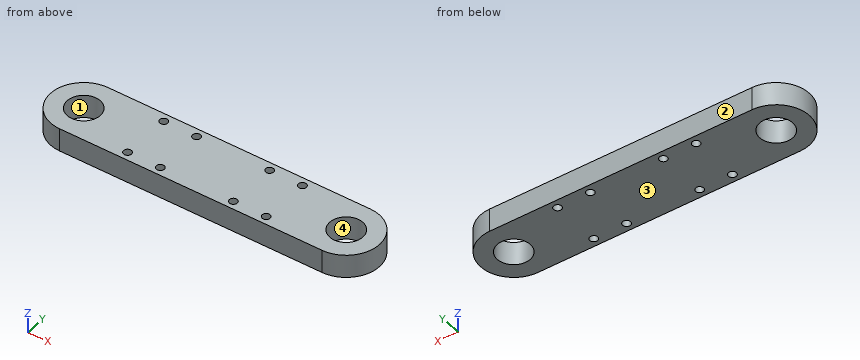
```python
from build123d import *

# Parameters (mm, degrees)
SKETCH_1_R          = 10
SKETCH_1_R_2        = 5
EXTRUDE_1_DEPTH     = 7
SKETCH_2_R          = 1.2
CUT_EXTRUDE_1_DEPTH = 10
CUT_EXTRUDE_START   = -10
SKETCH_3_R          = 5
CUT_EXTRUDE_2_DEPTH = 10
SKETCH_4_R          = 1.2
CUT_EXTRUDE_3_DEPTH = 10


with BuildPart() as part:
    # 草图1 → 凸台-拉伸1 (new body)
    # profile 1 of 2: a face of its own
    with BuildSketch(Plane.XY):
        Circle(SKETCH_1_R)
        Circle(SKETCH_1_R_2, mode=Mode.SUBTRACT)
    # profile 2 of 2: a face of its own
    with BuildSketch(Plane.XY):
        with BuildLine():
            Line((80, 10), (0, 10))
            ThreePointArc((0, 10), (7.071067812, 7.071067812), (10, 0))
            ThreePointArc((10, 0), (7.071067812, -7.071067812), (0, -10))
            Line((0, -10), (80, -10))
            ThreePointArc((80, -10), (90, 0), (80, 10))
        make_face()
    extrude(amount=EXTRUDE_1_DEPTH)

    # 草图2 → 切除-拉伸1 (cut)
    with BuildSketch(Plane(origin=(0, 0, 0), x_dir=(-1, 0, 0), z_dir=(0, 0, -1))):
        with Locations((-51.129038153, -7.5)):
            Circle(SKETCH_2_R)
        with Locations((-61.129038153, -7.5)):
            Circle(SKETCH_2_R)
        with Locations((-61.129038153, 7.5)):
            Circle(SKETCH_2_R)
        with Locations((-51.129038153, 7.5)):
            Circle(SKETCH_2_R)
    extrude(amount=-CUT_EXTRUDE_1_DEPTH, mode=Mode.SUBTRACT)

    # 草图3 → 切除-拉伸2 (cut)
    with BuildSketch(Plane.XY.offset(7).offset(CUT_EXTRUDE_START)):
        Circle(SKETCH_3_R)
        with Locations((80, 0)):
            Circle(SKETCH_3_R)
    extrude(amount=CUT_EXTRUDE_2_DEPTH, mode=Mode.SUBTRACT)

    # 草图4 → 切除-拉伸3 (cut)
    with BuildSketch(Plane.XY.offset(7).offset(CUT_EXTRUDE_START)):
        with Locations(Location((61.129038153, 7.5, 0), (0, 0, 180))):
            Circle(SKETCH_4_R)
        with Locations(Location((61.129038153, -7.5, 0), (0, 0, 180))):
            Circle(SKETCH_4_R)
        with Locations(Location((51.129038153, -7.5, 0), (0, 0, 180))):
            Circle(SKETCH_4_R)
        with Locations(Location((51.129038153, 7.5, 0), (0, 0, 180))):
            Circle(SKETCH_4_R)
        with Locations((28.870961847, 7.5)):
            Circle(SKETCH_4_R)
        with Locations((28.870961847, -7.5)):
            Circle(SKETCH_4_R)
        with Locations((18.870961847, -7.5)):
            Circle(SKETCH_4_R)
        with Locations((18.870961847, 7.5)):
            Circle(SKETCH_4_R)
    extrude(amount=CUT_EXTRUDE_3_DEPTH, mode=Mode.SUBTRACT)


solid = part.part
```
For this review, take the finished solid that the model builds, in its own axes (mm). Face numbers are marked on the shaded views. Coordinates: 2 decimals unless noted, no trailing zeros. Loops run counter-clockwise (first coordinate to the right, second up) from the corner with the lowest first, then second, coordinate; pieces in that order, holes last. Notation, with made-up numbers: (32, 48) - (50, 48) arc R23 cw to (50, 87) - close; hole circle Ø2 at (5.25, 10). An arc over 180 degrees is marked (long way). Use one line per item in the form item = value. Start each with the question number.
1) Draft analysis for pull direction Y (two halves, no side actions). For the marked faces 1, 2, 3 and 4, state which applies: released by +Y, released by -Y, zero draft, split by the parting line, or undercut.
2) To check wall thickness, follow probe 1 along X at (y, z) = (-0.25, 3); probe 2 along X at (y, z) = (-3, 0.75); probe 3 along X at (y, z) = (6.5, 1.75). State the ranges of each line that lie inside material, in increasing order. Write a range as from..to.
3) Take a section at B-B (z = 2.25). State how many separate pieces and enclosed holes the cut face has, plus the area to 3 significant figures.
4) Take a section at A-A (y = 0). State the section outline as (x, z) points.
5) Take a section at C-C (y = -7.5). State the section outline as (x, z) points, plus the area to 3 significant figures.
6) For pin 1 (4 mm diameter, centred on x = 51.13, y = 7.5, fed in from +Z), flat-tipped, find the tip position at first contact; note if it passes through.
From the geometry:
q1.face_1 = undercut
q1.face_2 = released by +Y
q1.face_3 = zero draft
q1.face_4 = undercut
q2.probe_1 = -10..-4.99, 4.99..75.01, 84.99..90
q2.probe_2 = -9.54..-4, 4..76, 84..89.54
q2.probe_3 = -7.6..18.21, 19.53..28.21, 29.53..50.47, 51.79..60.47, 61.79..87.6
q3.separate_pieces = 1
q3.enclosed_holes = 10
q3.area = 1,720 mm2
q4.outline = (-10, 0) - (-5, 0) - (-5, 7) - (-10, 7) - close; (5, 0) - (75, 0) - (75, 7) - (5, 7) - close; (85, 0) - (90, 0) - (90, 7) - (85, 7) - close
q5.outline = (-6.61, 0) - (17.67, 0) - (17.67, 7) - (-6.61, 7) - close; (20.07, 0) - (27.67, 0) - (27.67, 7) - (20.07, 7) - close; (30.07, 0) - (49.93, 0) - (49.93, 7) - (30.07, 7) - close; (52.33, 0) - (59.93, 0) - (59.93, 7) - (52.33, 7) - close; (62.33, 0) - (86.61, 0) - (86.61, 7) - (62.33, 7) - close
q5.area = 585 mm2
q6.pin_1 = 7
